from build123d import *

# Parameters (mm, degrees)
SKETCH1_W           = 45
SKETCH1_H           = 6
SKETCH1_W_2         = 6
BOSS_EXTRUDE1_DEPTH = 4
SKETCH2_R           = 1.8
CUT_EXTRUDE1_DEPTH  = 52.778373864
FILLET2_SIZE        = 6
FILLET3_R           = 2.5


with BuildPart() as part:
    # Sketch1 → Boss-Extrude1 (new body)
    with BuildSketch(Plane.XY):
        with Locations((-22.5, -3)):
            Rectangle(SKETCH1_W, SKETCH1_H)
        Polygon((-45, 0), (-39, 0), (-39, 8), (-45, 8), (-45, 2), align=None)
        with Locations((-48, 5)):
            Rectangle(SKETCH1_W_2, SKETCH1_H)
    extrude(amount=BOSS_EXTRUDE1_DEPTH)

    # Sketch2 → Cut-Extrude1 (cut, through all)
    with BuildSketch(Plane(origin=(0, 0, 0), x_dir=(-1, 0, 0), z_dir=(0, 0, -1))):
        with Locations((3, -3)):
            Circle(SKETCH2_R)
        with Locations((37, -3)):
            Circle(SKETCH2_R)
        with Locations((48, 5)):
            Circle(SKETCH2_R)
    extrude(amount=-CUT_EXTRUDE1_DEPTH, mode=Mode.SUBTRACT)

    # Fillet2
    # a fillet whose section is not a circle: 6 mm, written as the material it takes off along each edge
    with BuildSketch(Plane(origin=(-45, -6, -15), x_dir=(1, 0, 0), z_dir=(0, 0, 1))) as fillet2_piece_1:
        with BuildLine():
            Bezier((FILLET2_SIZE, 0), (0, 0), (0, FILLET2_SIZE), weights=[1, 0.428571429, 1])
            Line((0, FILLET2_SIZE), (0, 0))
            Line((0, 0), (FILLET2_SIZE, 0))
        make_face()
    extrude(amount=34, mode=Mode.SUBTRACT)
    with BuildSketch(Plane(origin=(-39, 8, -15), x_dir=(0, -1, 0), z_dir=(0, 0, 1))) as fillet2_piece_2:
        with BuildLine():
            Bezier((FILLET2_SIZE, 0), (0, 0), (0, -FILLET2_SIZE), weights=[1, 0.428571429, 1])
            Line((0, -FILLET2_SIZE), (0, 0))
            Line((0, 0), (FILLET2_SIZE, 0))
        make_face()
    extrude(amount=34, mode=Mode.SUBTRACT)

    # Fillet3
    fillet3_edges = [part.edges().sort_by_distance(p)[0] for p in [
        (-51, 8, 2),
        (-51, 2, 2),
        (-45, 2, 2),
        (-39, 0, 2),
        (0, 0, 2),
        (0, -6, 2),
    ]]
    fillet(fillet3_edges, radius=FILLET3_R)


solid = part.part
Geometry check sheet. Reference: the model listing, model coordinates, mm. A direction names the side the tool comes from. Round coordinates to 2 decimals unless told otherwise and drop trailing zeros. Loops run counter-clockwise (first coordinate to the right, second up) from the corner with the lowest first, then second, coordinate; pieces in that order, holes last. Notation, with made-up numbers: (-37, -5.5) -> (-28, -5.5) arc R18 cw to (-28, 9.5) -> close; hole circle Ø2 at (-39, 9). An arc over 180 degrees is marked (long way). Answer as a JSON object with one key per item and string values. Group by question number.
Item 1: Release check for a two-part mould opening along Y. For faces 4 (the face through (-4.717, -2.459, 1.972)), 5 (the face through (-47, 8, 2)), 6 (the face through (-26, -2, 4)) record: pulls with the +Y half, pulls with the -Y half, needs draft (parallel to the pull), parting line crosses it, or undercut.
Item 2: Cross-section at B-B, the plane x = -17.5. Record the cut outline in (y, z), plus the area to 3 significant figures.
Item 3: Set-up check for faces 1 (the face through (-48, 2, 2)), 2 (the face through (-20, 0, 2)), 3 (the face through (-51, 5, 2)): record each of +Z, -Z, +X, -X, +Y, -Y from which the full face is reachable in a straight line by a thin tool's end or side.
Item 4: Cross-section at C-C, the plane z = 0.8. Count the separate pieces of the cut face and the enclosed holes in it, plus the area to 3 significant figures.
Item 5: Cross-section at A-A, the plane x = -3. Record the cut outline in (y, z).
Item 6: Depth check by flat-ended pin: pin 1 Ø2 at (x, z) = (-22, 2) entering from +Y; pin 2 Ø1.1 at (x, z) = (-48, 1.5) entering from -Y; pin 3 Ø1 at (y, z) = (2, 2) entering from +X. Enter the tip coordinate at first touch or a pass-through.
Item 7: Thickness scan on line 1 along Y through (x, z) = (-48, 2.2); line 2 along X through (y, z) = (-3.5, 2.75); line 3 along Y through (x, z) = (-3, 1.45). Record the ranges inside material, lowest first.
Determined:
{
 "1": {"face 4": "undercut", "face 5": "pulls with the +Y half", "face 6": "needs draft"},
 "2": {"outline": "(-6, 0) -> (0, 0) -> (0, 4) -> (-6, 4) -> close", "area": "24.0 mm²"},
 "3": {"face 1": "+Z, -Z, -X, -Y", "face 2": "+Z, -Z, +X, +Y", "face 3": "+Z, -Z, -X, +Y, -Y"},
 "4": {"separate pieces": "1", "enclosed holes": "3", "area": "300 mm²"},
 "5": {"outline": "(-6, 0) -> (-4.8, 0) -> (-4.8, 4) -> (-6, 4) -> close; (-1.2, 0) -> (0, 0) -> (0, 4) -> (-1.2, 4) -> close"},
 "6": {"pin 1": "stops at y = 0", "pin 2": "stops at y = 2", "pin 3": "stops at x = -38.82"},
 "7": {"line 1": "y = 2 to 3.2, 6.8 to 8", "line 2": "x = -43.28 to -38.73, -35.27 to -4.73, -1.27 to 0", "line 3": "y = -6 to -4.8, -1.2 to 0"}
}
